Geometry check sheet. Reference: the model listing, model coordinates, mm. Face numbers are marked on the shaded views. A direction names the side the tool comes from. Give positions to 0.01 mm unless a question says otherwise; leave off trailing zeros. Write each loop counter-clockwise with the first axis right and the second up, starting at its lowest first coordinate (ties: lowest second). Pieces come first, ordered by that corner, then holes.
(1) Cross-section at C-C (x = 8.5). Record the boundary of the cut face in (y, z).
(2) Mould release check, pull along Y, two halves, no side actions. Record for the marked faces 4, 5, 6 and 7: +Y half, -Y half, draft (parallel to the pull), parting line (faces both ways), or undercut.
(3) Thickness scan on line 1 along Z through (x, y) = (0, -6.5); line 2 along Y through (x, z) = (7.5, 33); line 3 along X through (y, z) = (-8.5, 4). Record the ranges inside material, lowest first.
(4) Cross-section at A-A (z = 39). Record the boundary of the cut face in (x, y), and give its area (3 significant figures).
(5) Tool access check on the marked faces 1, 2 and 3. Record the directions out of +Z, -Z, +X, -X, +Y, -Y that give a thin tool (end or side, any length) a straight path to the whole face; none if there is none.
(6) Cross-section at B-B (y = 0). Record the boundary of the cut face in (x, z), and give its area (3 significant figures).
(7) Depth check by flat-ended pin: P1, Ø0.9, axis at x = -0.5, z = 4, coming from the +Y side; P2, Ø6, axis at y = -12.5, z = 6.5, coming from the +X side; P3, Ø0.9, axis at x = -0.5, z = 3, coming from the -Y side. Enter the tip coordinate at first touch or a pass-through.
(8) Cross-section at D-D (z = 26.5). Record the boundary of the cut face in (x, y).
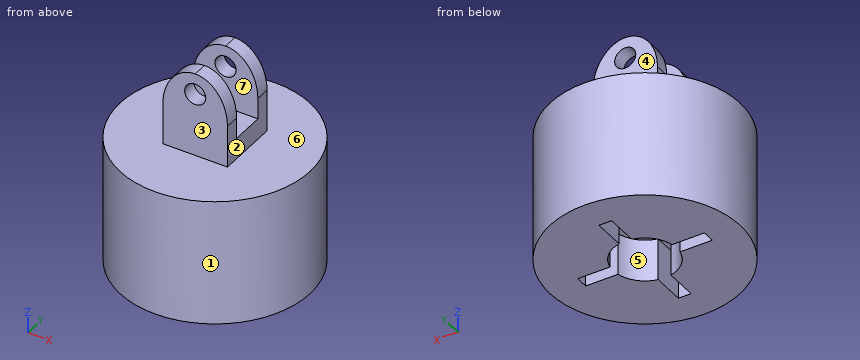
```python
from build123d import *

# Parameters (mm, degrees)
SKETCH1_R           = 22.5
BOSS_EXTRUDE1_DEPTH = 30
SKETCH2_R           = 7.5
SKETCH2_W           = 3
SKETCH2_H           = 30
SKETCH2_W_2         = 30
SKETCH2_H_2         = 3
CUT_EXTRUDE1_DEPTH  = 10
SKETCH3_W           = 15.299534312
SKETCH3_H           = 14.93812799
BOSS_EXTRUDE2_DEPTH = 20
CUT_EXTRUDE2_DEPTH  = 20
SKETCH5_R           = 2.5
CUT_EXTRUDE4_DEPTH  = 20


with BuildPart() as part:
    # Sketch1 → Boss-Extrude1 (new body)
    with BuildSketch(Plane.XY):
        Circle(SKETCH1_R)
    extrude(amount=BOSS_EXTRUDE1_DEPTH)

    # Sketch2 → Cut-Extrude1 (cut)
    with BuildSketch(Plane(origin=(0, 0, 0), x_dir=(-1, 0, 0), z_dir=(0, 0, -1))):
        Circle(SKETCH2_R)
        Rectangle(SKETCH2_W, SKETCH2_H)
        Rectangle(SKETCH2_W_2, SKETCH2_H_2)
    extrude(amount=-CUT_EXTRUDE1_DEPTH, mode=Mode.SUBTRACT)

    # Sketch3 → Boss-Extrude2 (add)
    with BuildSketch(Plane.XY.offset(30)):
        Rectangle(SKETCH3_W, SKETCH3_H)
    extrude(amount=BOSS_EXTRUDE2_DEPTH)

    # Sketch4 → Cut-Extrude2 (cut)
    with BuildSketch(Plane.ZY.offset(7.649767156)):
        Polygon((40, 4), (50, 4), (50, 0), (50, -4), (40, -4), (35, -4), (35, 4), align=None)
    extrude(amount=-CUT_EXTRUDE2_DEPTH, mode=Mode.SUBTRACT)

    # Sketch5 → Cut-Extrude4 (cut)
    with BuildSketch(Plane(origin=(0, 7.469063995, 0), x_dir=(1, 0, 0), z_dir=(0, 1, 0))):
        with Locations((0, -45)):
            Circle(SKETCH5_R)
        with BuildLine():
            Line((7.649767156, -50), (7.649767156, -40))
            add(Edge.make_bspline(
                [(0, -50), (7.649767156, -50), (7.649767156, -40)],
                knots=[3.141592654, 3.141592654, 3.141592654, 4.71238898, 4.71238898, 4.71238898], degree=2, weights=[1, 0.707106781, 1]))
            Line((0, -50), (7.649767156, -50))
        make_face()
        with BuildLine():
            Line((-7.649767156, -50), (0, -50))
            add(Edge.make_bspline(
                [(-7.649767156, -40), (-7.649767156, -50), (0, -50)],
                knots=[1.570796327, 1.570796327, 1.570796327, 3.141592654, 3.141592654, 3.141592654], degree=2, weights=[1, 0.707106781, 1]))
            Line((-7.649767156, -40), (-7.649767156, -50))
        make_face()
    extrude(amount=-CUT_EXTRUDE4_DEPTH, mode=Mode.SUBTRACT)


solid = part.part
```
Reply:
1. outline: (-20.83, 0) - (-1.5, 0) - (-1.5, 10) - (1.5, 10) - (1.5, 0) - (20.83, 0) - (20.83, 30) - (-20.83, 30) - close
2. face 4: +Y half
2. face 5: undercut
2. face 6: draft
2. face 7: undercut
3. line 1: z = 10 to 42.5, 47.5 to 50
3. line 2: y = -7.47 to 7.47
3. line 3: x = -20.83 to -1.5, 1.5 to 20.83
4. outline: (-7.65, -7.47) - (7.65, -7.47) - (7.65, -4) - (-7.65, -4) - close; (-7.65, 4) - (7.65, 4) - (7.65, 7.47) - (-7.65, 7.47) - close
4. area: 106 mm2
5. face 1: +Z, -Z
5. face 2: +Z, +X, +Y, -Y
5. face 3: +Z, +X, -X, -Y
6. outline: (-22.5, 0) - (-15, 0) - (-15, 10) - (15, 10) - (15, 0) - (22.5, 0) - (22.5, 30) - (7.65, 30) - (7.65, 35) - (-7.65, 35) - (-7.65, 30) - (-22.5, 30) - close
6. area: 1,130 mm2
7. P1: stops at y = 22.5
7. P2: stops at x = 20.4
7. P3: stops at y = -22.5
8. outline: circle Ø45 at (0, 0)
